Autodesk Inventor part; units mm, degrees
ref_plane "YZ Plane" through (0, 0, 0) normal (1, 0, 0) x (0, 1, 0)
ref_plane "XZ Plane" through (0, 0, 0) normal (0, 1, 0) x (-1, 0, 0)
ref_plane "XY Plane" through (0, 0, 0) normal (0, 0, 1) x (1, 0, 0)
sketch "Sketch1" plane through (0, 0, 0) normal (0, 0, 1) x (1, 0, 0)
  circle A0 centre (-78.0974, 78.0974) radius 31.75
  circle A1 centre (-78.0974, 78.0974) radius 38.1
  dimension "d0" = 76.2
extrude "Extrusion1" add sketch "Sketch1" along normal blind 6.35 contours A0 | A1
extrude "Extrusion2" add sketch "Sketch1" against normal blind 3.175 contours A0
sketch "Sketch3" plane through (-78.0974, 78.0974, -3.175) normal (0, 0, -1) x (-1, 0, 0)
  circle A0 centre (0, 0) radius 31.75
  circle A1 centre (0, 0) radius 34.925
  dimension "d5" = 69.85
extrude "Extrusion3" add sketch "Sketch3" along normal blind 3.175 contours A0 | A1
fillet "Fillet1" radius 3.175 1 edges at (-116.1974, 78.0974, 6.35)
sketch "Sketch4" plane through (-78.0974, 78.0974, 6.35) normal (0, 0, 1) x (1, 0, 0)
  circle A0 centre (0, 0) radius 34.925
  circle A1 centre (-19.05, 0) radius 6.9166
  circle A2 centre (19.05, 0) radius 6.9166
  dimension "d12" = 19.05
  dimension "d13" = 38.1
extrude "Extrusion4" cut sketch "Sketch4" against normal through all contours A1 | A2
equation "\"d13\" = 2 * d12"
properties part number "INSULATION-GASKET-2" material "Phenolic"
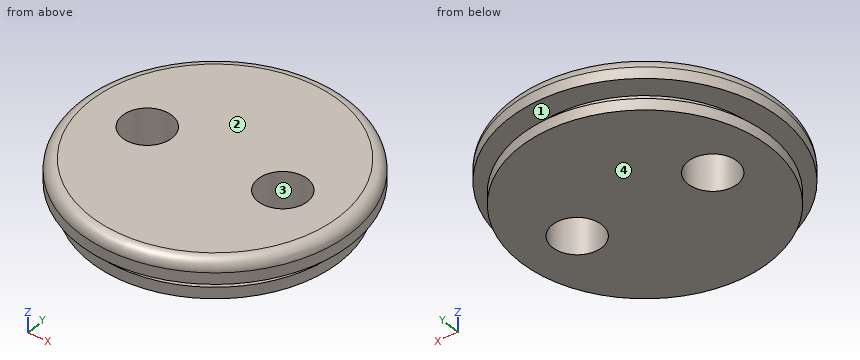
Could you check a few things on this model? Use its own coordinates, in mm. Face numbers are marked on the shaded views. A direction names the side the tool comes from. Give positions to 0.01 mm unless a question says otherwise; leave off trailing zeros. Order: outer loops, then holes, each group sorted by start corner. A loop starts at its lowest first (then second) coordinate and runs counter-clockwise, first axis right, second up.
1. For the marked faces 1 and 2, which set-ups out of +Z, -Z, +X, -X, +Y, -Y let a thin tool reach every point of the face, with its end or its side?
2. I need wall thicknesses on L1, parallel to X at y = 80, z = -2; L2, parallel to X at y = 81.5, z = -3; L3, parallel to Y at x = -78, z = -4.5. Which ranges of each line are inside material? Lowest first, please.
3. Suppose I cut it at B-B (y = 83.5). Give the number of separate pieces and of enclosed holes in the cut face, plus the area to 3 significant figures.
4. We'd pull the mould along Y, two halves only. Please class the marked faces 3 and 4: pulls with the +Y half, pulls with the -Y half, needs draft (parallel to the pull), parting line crosses it, or undercut.
5. Will these pins go through, and if not, where does the flat tip stop? P1, Ø1.5, axis at y = 74, z = -2.5, coming from the +X side; P2, Ø18, axis at x = -97.15, y = 78.1, coming from the +Z side; P3, Ø1, axis at x = -70.5, z = -4, coming from the -Y side; P4, Ø6, axis at y = 52, z = -1, coming from the +X side.
6. Suppose I cut it at A-A (z = -5). List the corners of the cut face in (x, y) for me (3 decimals).
Solved:
1. face 1: none
1. face 2: +Z, +X, -X, +Y, -Y
2. L1: x = -109.79 to -103.8, -90.5 to -65.7, -52.4 to -46.4
2. L2: x = -109.66 to -103.17, -91.13 to -65.07, -53.03 to -46.53
2. L3: y = 43.17 to 113.02
3. separate pieces: 3
3. enclosed holes: 0
3. area: 673 mm2
4. face 3: undercut
4. face 4: needs draft
5. P1: stops at x = -43.38
5. P2: stops at z = 6.35
5. P3: stops at y = 43.9
5. P4: stops at x = -47.93
6. outline: circle Ø69.85 at (-78.097, 78.097); hole circle Ø13.833 at (-97.147, 78.097); hole circle Ø13.833 at (-59.047, 78.097)
